Part model, mm, in its own coordinate system. Face numbers are marked on the shaded views. A direction names the side the tool comes from. Coordinates: 2 decimals unless noted, no trailing zeros. Loops run counter-clockwise (first coordinate to the right, second up) from the corner with the lowest first, then second, coordinate; pieces in that order, holes last. Notation, with made-up numbers: M 69.25,60 L 95.25,60 A3 cw 95.25,65 Z; hole C -18.75,43.5 d1. An arc over 180 degrees is marked long. Use a Markdown table: item, result. Add a question column.
1) Tool access for the marked faces 1, 2 and 3: list every direction of +Z, -Z, +X, -X, +Y, -Y with a clear straight run to the whole face (end or side of a thin tool).
2) Wall check: probe 1 along Y at (x, z) = (-13, 3); probe 2 along Z at (x, y) = (-9, 46); probe 3 along X at (y, z) = (41.5, 0). Give the ranges that are in metal, low to high. Write a range as from..to.
3) Band-saw the part on C-C (y = 26.5). List the corners of the cut face in (x, z), plus the area to 3 significant figures.
4) Pull direction X, two halves, no side cores. Call the marked faces 4, 5 and 6: released by +X, released by -X, zero draft, split by the parting line, or undercut.
5) Band-saw the part on A-A (x = 1). List the corners of the cut face in (y, z).
6) Pin check, flat tips, straight feed: pin 1 Ø3 at (x, y) = (-13.5, 49) entering from -Z; pin 2 Ø2 at (y, z) = (13.5, 1.5) entering from +X; pin 3 Ø5 at (x, y) = (10, 16.5) entering from -Z. Stop position of each tip, or through.
7) Band-saw the part on B-B (y = 13). List the corners of the cut face in (x, z), plus the area to 3 significant figures.
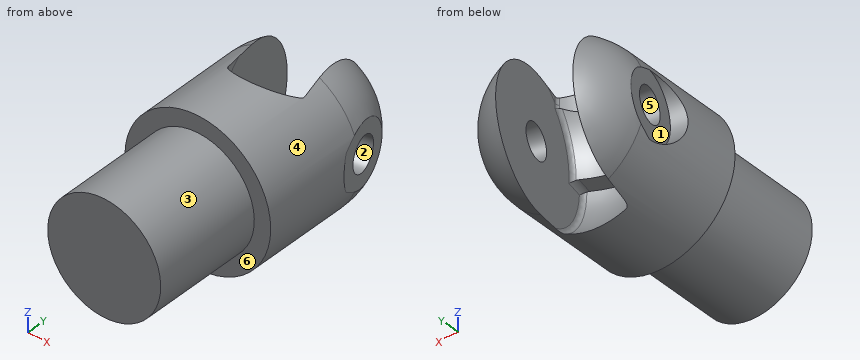
from build123d import *

# Parameters (mm, degrees)
SKETCH1_R                     = 12.9921
BOSS_EXTRUDE1_DEPTH           = 25.4
CUT_EXTRUDE1_DEPTH            = 104.344307451
CUT_EXTRUDE1_DEPTH_BACK       = 104.344307451
SKETCH3_R                     = 3.81
CUT_REVOLVE10_ANGLE           = 180
CUT_REVOLVE10_OTHER_WAY_ANGLE = 90
CUT_EXTRUDE4_DEPTH            = 32.004
FILLET1_R                     = 1.27
SKETCH15_R                    = 7.62
CUT_EXTRUDE5_DEPTH            = 10.16


with BuildPart() as part:
    # Sketch1 → Boss-Extrude1 (new body)
    with BuildSketch(Plane(origin=(0, 0, 0), x_dir=(1, 0, 0), z_dir=(0, 1, 0))):
        with Locations(Location((0, 0, 0), (0, 0, 270))):
            Circle(SKETCH1_R)
    extrude(amount=BOSS_EXTRUDE1_DEPTH)

    # Sketch2 → Revolve1 (revolve)
    with BuildSketch(Plane(origin=(0, 0, 0), x_dir=(0, 0, -1), z_dir=(1, 0, 0))):
        with BuildLine():
            Line((-16.764, 25.4), (-16.764, 49.53))
            ThreePointArc((-16.764, 49.53), (-11.85393808, 61.38393808), (0, 66.294))
            Line((0, 66.294), (0, 25.4))
            Line((0, 25.4), (-16.764, 25.4))
        make_face()
    revolve(axis=Axis((0, 25.4, 0), (0, 1, 0)))

    # Sketch3 → Cut-Extrude1 (cut, two sides: drawn at the far end of the back side and taken through both)
    with BuildSketch(Plane(origin=(-10.366451402, 98.300319395, 0), x_dir=(0, 0, -1), z_dir=(-0.9781476007338062, -0.20791169081775643, 0)).offset(-CUT_EXTRUDE1_DEPTH_BACK)):
        with Locations(Location((0, 49.859877342, 0), (0, 0, 65.612599739))):
            Circle(SKETCH3_R)
    extrude(amount=CUT_EXTRUDE1_DEPTH + CUT_EXTRUDE1_DEPTH_BACK, mode=Mode.SUBTRACT)

    # Sketch11 → Cut-Revolve10 (revolve, cut)
    with BuildSketch(Plane.XY):
        with BuildLine():
            Line((-7.701934208, 47.892903347), (-11.162976054, 64.175825024))
            ThreePointArc((-11.162976054, 64.175825024), (-4.101170935, 67.482510185), (3.695979409, 67.570287171))
            Line((3.695979409, 67.570287171), (7.205035227, 51.061477515))
            Line((7.205035227, 51.061477515), (-7.701934208, 47.892903347))
        make_face()
    revolve(axis=Axis((17.487516564, 53.247086393, 0), (-0.9781476007338064, -0.2079116908177564, 0)), revolution_arc=CUT_REVOLVE10_ANGLE, mode=Mode.SUBTRACT)

    # Sketch11 → Cut-Revolve10 other way (revolve, cut)
    with BuildSketch(Plane.XY):
        with BuildLine():
            Line((-7.701934208, 47.892903347), (-11.162976054, 64.175825024))
            ThreePointArc((-11.162976054, 64.175825024), (-4.101170935, 67.482510185), (3.695979409, 67.570287171))
            Line((3.695979409, 67.570287171), (7.205035227, 51.061477515))
            Line((7.205035227, 51.061477515), (-7.701934208, 47.892903347))
        make_face()
    revolve(axis=Axis((17.487516564, 53.247086393, 0), (0.9781476007338064, 0.2079116908177564, 0)), revolution_arc=CUT_REVOLVE10_OTHER_WAY_ANGLE, mode=Mode.SUBTRACT)

    # Sketch13 → Cut-Revolve11 (revolve, cut)
    with BuildSketch(Plane.XY):
        with BuildLine():
            Line((-8.49407775, 51.619645705), (6.412891685, 54.788219873))
            Line((6.412891685, 54.788219873), (2.927360083, 71.186356794))
            ThreePointArc((2.927360083, 71.186356794), (-4.869286819, 71.216520857), (-11.979609352, 68.017782626))
            Line((-11.979609352, 68.017782626), (-8.49407775, 51.619645705))
        make_face()
    revolve(axis=Axis((-8.49407775, 51.619645705, 0), (0.9781476007338064, 0.20791169081775632, 0)), mode=Mode.SUBTRACT)

    # Sketch14 → Cut-Extrude4 (cut)
    with BuildSketch(Plane.XY):
        with BuildLine():
            Line((-7.701934208, 47.892903347), (-6.149656223, 40.590009601))
            ThreePointArc((-6.149656223, 40.590009601), (1.969552427, 39.042311826), (8.757313212, 43.758583769))
            Line((8.757313212, 43.758583769), (7.205035227, 51.061477515))
            Line((7.205035227, 51.061477515), (-7.701934208, 47.892903347))
        make_face()
    extrude(amount=CUT_EXTRUDE4_DEPTH, mode=Mode.SUBTRACT)

    # Fillet1
    fillet1_edges = [part.edges().sort_by_distance(p)[0] for p in [
        (-4.840027967, 34.428693074, -9.361457334),
        (-4.624719256, 33.415745227, 0),
        (-5.306564153, 36.623573262, 6.782727573),
        (9.600405282, 39.79214743, 6.782727573),
        (-6.149656223, 40.590009601, 14.000445211),
        (8.757313212, 43.758583769, 13.350191985),
        (10.306257166, 36.471375406, 0),
        (10.298585015, 36.507470038, -7.966497668),
    ]]
    fillet(fillet1_edges, radius=FILLET1_R)

    # Sketch15 → Cut-Extrude5 (cut)
    with BuildSketch(Plane(origin=(-4.834136469, -1.027527427, 0), x_dir=(0, 0, -1), z_dir=(-0.9781476007338062, -0.20791169081775643, 0))):
        with Locations((0, -48.447650664)):
            Circle(SKETCH15_R)
    cut_extrude5 = extrude(amount=CUT_EXTRUDE5_DEPTH, mode=Mode.SUBTRACT)

    # Mirror1: Cut-Extrude5 across plane
    add(cut_extrude5.mirror(Plane(origin=(10.072832966, 2.141046741, 0), x_dir=(0, 0, 1), z_dir=(-0.9781476007338062, -0.20791169081775643, 0))), mode=Mode.SUBTRACT)


solid = part.part
Entries:
| question | item | result |
|---|---|---|
| 1 | face 1 | -X |
| 1 | face 2 | none |
| 1 | face 3 | -Y |
| 2 | probe 1 | 25.4..44.37, 49.17..59.68 |
| 2 | probe 2 | -14.14..-3.47, 3.47..14.14 |
| 2 | probe 3 | -13.87..-6.34, 9.24..16.76 |
| 3 | outline | C 0,0 d33.53 |
| 3 | area | 883 mm2 |
| 4 | face 4 | split by the parting line |
| 4 | face 5 | undercut |
| 4 | face 6 | zero draft |
| 5 | outline | M 0,-12.95 L 25.4,-12.95 L 25.4,-16.73 L 41.91,-16.73 A18.39 cw 31.14,0 L 34.9,0 A18.3 cw 38.88,11.39 L 38.88,16.73 L 25.4,16.73 L 25.4,12.95 L 0,12.95 Z |
| 6 | pin 1 | z = -11.71 |
| 6 | pin 2 | x = 12.98 |
| 6 | pin 3 | z = -10.61 |
| 7 | outline | C 0,0 d25.98 |
| 7 | area | 530 mm2 |
